Geometry check sheet. Reference: the model listing, model coordinates, mm. Coordinates: 2 decimals unless noted, no trailing zeros. Loops run counter-clockwise (first coordinate to the right, second up) from the corner with the lowest first, then second, coordinate; pieces in that order, holes last.
from build123d import *

# Parameters (mm, degrees)
SKETCH2_R          = 2.75
CUT_EXTRUDE1_DEPTH = 0.1
CUT_EXTRUDE2_DEPTH = 0.1
SKETCH4_W          = 0.3
SKETCH4_H          = 2.5
SKETCH5_W          = 0.3
SKETCH5_H          = 2.5
FILLET1_R          = 0.5


with BuildPart() as part:
    # Sketch1 → Revolve1 (revolve)
    with BuildSketch(Plane.XY):
        with BuildLine():
            Line((4, 11.5), (0, 11.5))
            Line((0, 11.5), (0, 0))
            Line((0, 0), (3.643923536, 0))
            ThreePointArc((3.643923536, 0), (3.925044146, 0.40653797), (3.851388969, 0.895288247))
            ThreePointArc((3.851388969, 0.895288247), (3.78355892, 1.057917503), (3.760416667, 1.232599004))
            Line((3.760416667, 1.232599004), (3.760416667, 1.642400996))
            ThreePointArc((3.760416667, 1.642400996), (3.791064683, 1.842850794), (3.880208333, 2.024984899))
            ThreePointArc((3.880208333, 2.024984899), (3.969351983, 2.207119004), (4, 2.407568802))
            Line((4, 2.407568802), (4, 11.5))
        make_face()
    revolve(axis=Axis((0, 11.5, 0), (0, -1, 0)))

    # Sketch2 → Cut-Extrude1 (cut)
    with BuildSketch(Plane(origin=(0, 11.5, 0), x_dir=(-1, 0, 0), z_dir=(0, 1, 0))):
        with Locations(Location((0, 0, 0), (0, 0, 270))):
            Circle(SKETCH2_R)
    extrude(amount=-CUT_EXTRUDE1_DEPTH, mode=Mode.SUBTRACT)

    # Sketch3 → Cut-Extrude2 (cut)
    with BuildSketch(Plane(origin=(0, 11.4, 0), x_dir=(-1, 0, 0), z_dir=(0, 1, 0))):
        Polygon((1.653472744, -1.932293167), (1.837973446, -1.757720858), (0.142645036, 0.03402539), (0.846678598, 2.398095985), (0.603244193, 2.470592124), (-0.10078937, 0.10652153), (-2.500151342, -0.465802817), (-2.441217638, -0.712871266), (-0.041855666, -0.14054692), align=None)
    extrude(amount=-CUT_EXTRUDE2_DEPTH, mode=Mode.SUBTRACT)

    # Sketch4 → Revolve2 (revolve)
    with BuildSketch(Plane(origin=(0, 0, 0), x_dir=(-1, 0, 0), z_dir=(0, 0, -1)), mode=Mode.PRIVATE) as revolve2_sk:
        with Locations((-1.9, -1.25)):
            Rectangle(SKETCH4_W, SKETCH4_H)
    revolve(revolve2_sk.sketch.rotate(Axis((1.75, -2.5, 0), (0, 1, 0)), 270), axis=Axis((1.75, -2.5, 0), (0, 1, 0)))

    # Sketch5 → Revolve3 (revolve)
    with BuildSketch(Plane(origin=(0, 0, 0), x_dir=(-1, 0, 0), z_dir=(0, 0, -1)), mode=Mode.PRIVATE) as revolve3_sk:
        with Locations((1.6, -1.25)):
            Rectangle(SKETCH5_W, SKETCH5_H)
    revolve(revolve3_sk.sketch.rotate(Axis((-1.75, -2.5, 0), (0, 1, 0)), 270), axis=Axis((-1.75, -2.5, 0), (0, 1, 0)))

    # Fillet1
    fillet1_edges = [part.edges().sort_by_distance(p)[0] for p in [
        (-4, 11.5, 0),
        (-3.643923536, 0, 0),
    ]]
    fillet(fillet1_edges, radius=FILLET1_R)


solid = part.part
1) Mould release check, pull along X, two halves, no side actions. Record for faces 1 (the cylindrical face through (-0.82, 1.44, -3.67)), 2 (the flat face through (0, 11.4, -1)), 3 (the flat face through (-3, 11.5, -1)): +X half, -X half, draft (parallel to the pull), parting line (faces both ways), or undercut.
Data:
face 1: parting line
face 2: undercut
face 3: draft
2) Material ranges on probe 1 along Y at (x, z) = (-0.5, -2.25); probe 2 along Y at (x, z) = (2.75, -1); probe 3 along Z at (x, y) = (0.25, 2), recorded low to high.
Data:
probe 1: y = 0 to 11.4
probe 2: y = 0 to 11.5
probe 3: z = -3.86 to 3.86
3) Section check B-B on y = 6.5. Record the cut outline in (x, z).
Data:
outline: circle Ø8 at (0, 0)
4) Section check A-A on y = -1. Record the cut outline in (x, z), and give its area (3 significant figures).
Data:
outline: circle Ø0.6 at (-1.75, 0); circle Ø0.6 at (1.75, 0)
area: 0.565 mm2
5) Depth check by flat-ended pin: pin 1 (1.6 mm diameter, centred on x = 0.5, z = 1, fed in from +Y); pin 2 (3 mm diameter, centred on x = 0, z = -3, fed in from -Y). Enter the tip coordinate at first touch or a pass-through.
Data:
pin 1: stops at y = 11.4
pin 2: stops at y = 0
